from build123d import *

# Parameters (mm, degrees)
ESQUISSE1_W        = 200
ESQUISSE1_H        = 180
ESQUISSE1_R        = 10
BOSS_EXTRU_1_DEPTH = 10
ESQUISSE3_R        = 10
BOSS_EXTRU_2_DEPTH = 50
ESQUISSE4_W        = 20
ESQUISSE4_H        = 10
BOSS_EXTRU_3_DEPTH = 10


with BuildPart() as part:
    # Esquisse1 → Boss.-Extru.1 (new body)
    with BuildSketch(Plane.XY):
        Rectangle(ESQUISSE1_W, ESQUISSE1_H)
        with Locations((-30, 0)):
            Circle(ESQUISSE1_R, mode=Mode.SUBTRACT)
    extrude(amount=BOSS_EXTRU_1_DEPTH)

    # Esquisse3 → Boss.-Extru.2 (add)
    with BuildSketch(Plane(origin=(0, 0, 0), x_dir=(-1, 0, 0), z_dir=(0, 0, -1))):
        with Locations((30, 0)):
            Circle(ESQUISSE3_R)
    extrude(amount=-BOSS_EXTRU_2_DEPTH)

    # Esquisse4 → Boss.-Extru.3 (add)
    with BuildSketch(Plane.XY.offset(10)):
        with Locations((-80, -20)):
            Rectangle(ESQUISSE4_W, ESQUISSE4_H)
        Polygon((-12.32233047, -38.890872965), (1.819805153, -53.033008589), (-5.251262658, -60.104076401), (-19.393398282, -45.961940777), align=None)
    extrude(amount=BOSS_EXTRU_3_DEPTH)


solid = part.part
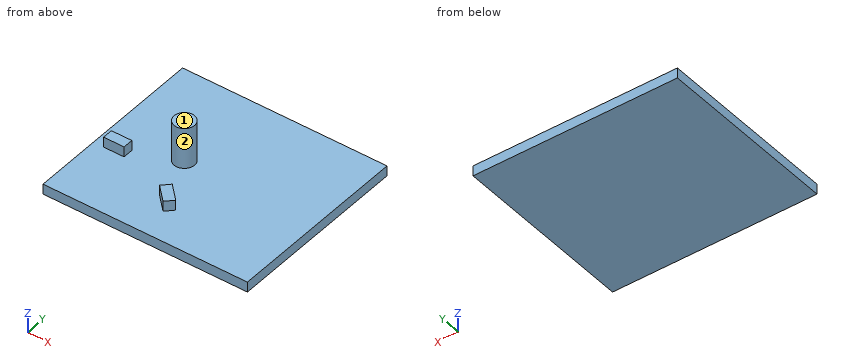
CAD build for the part. Positions are in the model's coordinates, mm. Face numbers are marked on the shaded views. A direction names the side the tool comes from. Coordinates: 2 decimals unless noted, no trailing zeros. Loops run counter-clockwise (first coordinate to the right, second up) from the corner with the lowest first, then second, coordinate; pieces in that order, holes last. Notation, with made-up numbers: (12.25, 23.5) - (38.25, 23.5) arc R33 cw to (38.25, 60.5) - close; hole circle Ø8 at (-24, 53.25). An arc over 180 degrees is marked (long way). Use one line per item in the form item = value. Start each with the question number.
1) Band-saw the part on D-D (y = -77.5). Give the cut face in (x, z).
2) Band-saw the part on B-B (x = -76). Give the cut face in (y, z).
3) Band-saw the part on C-C (z = 44). Give the cut face in (x, y), and give its area (3 significant figures).
4) Tool access for the marked faces 1 and 2: list every direction of +Z, -Z, +X, -X, +Y, -Y with a clear straight run to the whole face (end or side of a thin tool).
5) Drill centre lines: L1, parallel to Z at x = -6.5, y = -45; L2, parallel to Z at x = -84, y = 19; L3, parallel to Y at x = -4, z = 11. Where is each one in solid material? Low to high. Write a range as from..to.
6) Flat gauge pins, fed straight in: pin 1 (23.5 mm diameter, centred on x = -9.5, y = -52.5, fed in from +Z); pin 2 (5 mm diameter, centred on y = -39, z = 14.5, fed in from -X); pin 3 (5 mm diameter, centred on y = -53, z = 20.5, fed in from +X). Where does each tip first touch, or does it go through?
7) Band-saw the part on A-A (y = 0). Give the cut face in (x, z).
Check values:
q1.outline = (-100, 0) - (100, 0) - (100, 10) - (-100, 10) - close
q2.outline = (-90, 0) - (90, 0) - (90, 10) - (-15, 10) - (-15, 20) - (-25, 20) - (-25, 10) - (-90, 10) - close
q3.outline = circle Ø20 at (-30, 0)
q3.area = 314 mm2
q4.face_1 = +Z, +X, -X, +Y, -Y
q4.face_2 = +Z
q5.L1 = 0..20
q5.L2 = 0..10
q5.L3 = -58.85..-47.21
q6.pin_1 = 20
q6.pin_2 = -14.93
q6.pin_3 = 1.82
q7.outline = (-100, 0) - (100, 0) - (100, 10) - (-20, 10) - (-20, 50) - (-40, 50) - (-40, 10) - (-100, 10) - close
